Read the model definition and answer for the solid it produces. Units are mm, in the model's axes. Round coordinates to 2 decimals unless told otherwise and drop trailing zeros. Loops run counter-clockwise (first coordinate to the right, second up) from the corner with the lowest first, then second, coordinate; pieces in that order, holes last. Notation, with made-up numbers: M 10.5,69.25 L 48.5,69.25 A13 ccw 48.5,92.25 Z; hole C 83,9 d7. An arc over 180 degrees is marked long. Write each question's results on one line, items separated by ' | '.
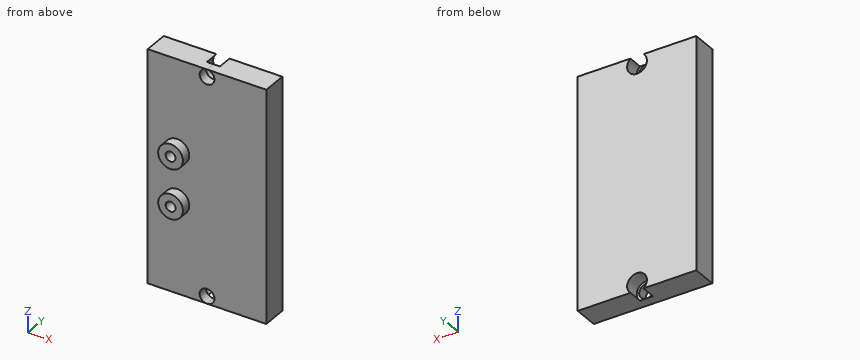
Autodesk Inventor part; units mm, degrees
ref_plane "YZ Plane" through (0, 0, 0) normal (1, 0, 0) x (0, 1, 0)
ref_plane "XZ Plane" through (0, 0, 0) normal (0, 1, 0) x (-1, 0, 0)
ref_plane "XY Plane" through (0, 0, 0) normal (0, 0, 1) x (1, 0, 0)
sketch "Sketch1" plane through (0, 0, 0) normal (0, 1, 0) x (-1, 0, 0)
  line L0 (12, 23.5) -> (-12, 23.5)
  line L1 (-12, 23.5) -> (-12, -23.5)
  line L2 (-12, -23.5) -> (12, -23.5)
  line L3 (12, -23.5) -> (12, 23.5)
  point P0 (0, 0)
  dimension "d0" = 12
  dimension "d1" = 12
  dimension "d2" = 23.5
  dimension "d3" = 23.5
extrude "Extrusion1" add sketch "Sketch1" along normal blind 5
sketch "Sketch2" plane through (0, 5, 0) normal (0, 1, 0) x (1, 0, 0)
  circle A0 centre (0, -22) radius 1.5
  circle A1 centre (0, 22) radius 1.5
  point P0 (0, 0)
  dimension "d6" = 3
  dimension "d7" = 3
  dimension "d8" = 22
  dimension "d9" = 22
  dimension "d10" = 0
  dimension "d11" = 0
extrude "Extrusion2" cut sketch "Sketch2" against normal up to surface (5 mm away)
sketch "Sketch4" plane through (0, 5, 0) normal (0, 1, 0) x (1, 0, 0)
  circle A0 centre (0, -22) radius 1.5
  circle A1 centre (0, 22) radius 1.5
  line L0 (-12, -23.5) -> (0, -23.5)
  line L1 (12, -23.5) -> (12, 23.5)
  line L2 (12, 23.5) -> (0, 23.5)
  line L3 (-12, 23.5) -> (-12, -23.5)
  circle A2 centre (0, -22) radius 2
  circle A3 centre (0, 22) radius 2
  line L4 (0, -23.5) -> (12, -23.5)
  line L5 (0, 23.5) -> (-12, 23.5)
  point P0 (0, 0)
  dimension "d14" = 4
  dimension "d15" = 4
extrude "Extrusion3" cut sketch "Sketch4" against normal blind 3 contours L0 A2 L4 | L4 A2 L0 | L5 L2 A3 | A3 L2 L5
sketch "Sketch5" plane through (0, 0, 0) normal (0, -1, 0) x (1, 0, 0)
  line L0 (6.9, -7.1144) -> (6.9, 7.2186)
  line L1 (6.9, 7.2186) -> (-8.137, 7.2)
  line L2 (-8.137, 7.2) -> (-8.104, -7.136)
  line L3 (-8.104, -7.136) -> (6.9, -7.1144)
  circle A0 centre (4.9456, 5.262) radius 0.4065
  circle A1 centre (4.9282, -4.9331) radius 0.4065
  circle A2 centre (4.9478, 2.722) radius 0.4065
  circle A3 centre (4.952, -2.358) radius 0.4065
  circle A4 centre (-6.0981, 4.9907) radius 1.5
  circle A5 centre (-6.0897, -5.0423) radius 1.5
  circle A6 centre (-6.0897, -5.0423) radius 1
  circle A7 centre (-6.0981, 4.9907) radius 1
  point P0 (0, 0)
  dimension "d24" = 1
  dimension "d25" = 1
extrude "Extrusion4" add sketch "Sketch5" along normal blind 0.01 contours A4 | A5 | A6 | A7
sketch "Sketch6" plane through (0, 0, 0) normal (0, -1, 0) x (1, 0, 0)
  circle A0 centre (-6.0981, 4.9907) radius 1.5
  circle A1 centre (-6.0897, -5.0423) radius 1.5
  circle A2 centre (0, 22) radius 1.5
  circle A3 centre (0, -22) radius 1.5
  line L0 (-12, 23.5) -> (0, 23.5)
  line L1 (-12, -23.5) -> (-12, 23.5)
  line L2 (12, -23.5) -> (0, -23.5)
  line L3 (12, 23.5) -> (12, -23.5)
  circle A4 centre (-6.0981, 4.9907) radius 2.5
  circle A5 centre (-6.0897, -5.0423) radius 2.5
  line L4 (0, -23.5) -> (-12, -23.5)
  line L5 (0, 23.5) -> (12, 23.5)
  point P0 (0, 0)
  dimension "d20" = 1
  dimension "d21" = 1
extrude "Extrusion5" add sketch "Sketch6" along normal blind 2 contours A4 | A5
sketch "Sketch7" plane through (-6.0897, -2, -5.0423) normal (0, -1, 0) x (1, 0, 0)
  circle A0 centre (0, 0) radius 1.5
  circle A1 centre (0, 0) radius 2.5
  circle A2 centre (-0.0084, 10.033) radius 1.5
  circle A3 centre (-0.0084, 10.033) radius 2.5
  circle A4 centre (0, 0) radius 1
  circle A5 centre (-0.0084, 10.033) radius 1
  point P0 (6.0897, 5.0423)
  dimension "d26" = 1
  dimension "d27" = 1
extrude "Extrusion6" add sketch "Sketch7" against normal blind 5 contours A0 | A2
properties part number "Bottom"
Item 1: The part is cut by section C-C (z = -19.5). Determine the outline of the cut face in (x, y), plus the area to 3 significant figures.
Outcome:
outline: M -12,0 L 12,0 L 12,5 L -12,5 Z | area: 120 mm2
Item 2: A flat-ended cylindrical pin translates along its axis: pin 1 (7 mm diameter, centred on x = -1, z = 1.5, fed in from -Y). Find the tip coordinate at first contact, or state that the pin passes through.
Outcome:
pin 1: stops at y = 0
Item 3: Straight lines are drawn through the part: line 1 (X direction, y = 0.9, z = 22); line 2 (Y direction, x = 0.25, z = -3.5); line 3 (Z direction, x = 0, y = 2.8). For each, find the intervals that lie inside material, in ascending order.
Outcome:
line 1: x = -12 to -1.5, 1.5 to 12 | line 2: y = 0 to 5 | line 3: z = -20 to 20
Item 4: The part is cut by section D-D (y = -1). Determine the outline of the cut face in (x, z), plus the area to 3 significant figures.
Outcome:
outline: C -6.1,4.99 d5; C -6.09,-5.04 d5; hole C -6.1,4.99 d2; hole C -6.09,-5.04 d2 | area: 33.0 mm2
Item 5: The part is cut by section B-B (y = 4.5). Determine the outline of the cut face in (x, z), plus the area to 3 significant figures.
Outcome:
outline: M -12,-23.5 L -1.32,-23.5 A2 cw long 1.32,-23.5 L 12,-23.5 L 12,23.5 L 1.32,23.5 A2 cw long -1.32,23.5 L -12,23.5 Z | area: 1,100 mm2
Item 6: The part is cut by section A-A (x = -0.5). Determine the outline of the cut face in (y, z), plus the area to 3 significant figures.
Outcome:
outline: M 0,-23.5 L 2,-23.5 L 2,-23.41 L 0,-23.41 Z; M 0,-20.59 L 2,-20.59 L 2,-20.06 L 5,-20.06 L 5,20.06 L 2,20.06 L 2,20.59 L 0,20.59 Z; M 0,23.41 L 2,23.41 L 2,23.5 L 0,23.5 Z | area: 203 mm2
